from build123d import *

# Parameters (mm, degrees)
F0_R     = 3.175
F0_W     = 1.2134287943
F0_H     = 4.4488144882
F1_DEPTH = 3.048


with BuildPart() as f1:
    # F0 (on Front) → F1 (new body)
    with BuildSketch(Plane.XZ):
        with BuildLine():
            ThreePointArc((44.7334821429, -7.9324362036), (50.1620069047, -5.5115227815), (52.3875, 0))
            ThreePointArc((52.3875, 0), (50.1620069047, 5.5115227815), (44.7334821429, 7.9324362036))
            ThreePointArc((44.7334821429, 7.9324362036), (36.5125, 0), (44.7334821429, -7.9324362036))
        make_face()
        with Locations((44.45, 0)):
            Circle(F0_R, mode=Mode.SUBTRACT)
        with BuildLine():
            ThreePointArc((44.7334821429, -7.9324362036), (36.5125, 0), (44.7334821429, 7.9324362036))
            Line((44.7334821429, 7.9324362036), (18.9676000005, 8.8532337108))
            ThreePointArc((18.9676000005, 8.8532337108), (13.2611998974, 11.5713591498), (11.3411865923, 17.5933818124))
            Line((11.3411865923, 17.5933818124), (15.7954255641, 61.9125))
            ThreePointArc((15.7954255641, 61.9125), (0, 47.625), (-15.7954255641, 61.9125))
            Line((-15.7954255641, 61.9125), (-9.4772553384, -0.9525))
            ThreePointArc((-9.4772553384, -0.9525), (-0.4768479324, 9.5130563464), (9.525, 0))
            ThreePointArc((9.525, 0), (6.8544082857, -6.6138273378), (0.3401785714, -9.5189234444))
            Line((0.3401785714, -9.5189234444), (44.7334821429, -7.9324362036))
        make_face()
        with BuildLine():
            add(Edge.make_bspline(
                [(-4.1992530573, 32.2494809549), (-4.5608624776, 32.1718113259), (-5.0829042464, 32.1718113259)],
                knots=[0, 0, 0, 1, 1, 1], degree=2))
            add(Edge.make_bspline(
                [(-5.0829042464, 32.1718113259), (-6.156273054, 32.1718113259), (-6.7610775422, 32.7651563606)],
                knots=[0, 0, 0, 1, 1, 1], degree=2))
            add(Edge.make_bspline(
                [(-6.7610775422, 32.7651563606), (-7.3658820304, 33.3585013954), (-7.3658820304, 34.444602929)],
                knots=[0, 0, 0, 1, 1, 1], degree=2))
            add(Edge.make_bspline(
                [(-7.3658820304, 34.444602929), (-7.3658820304, 35.5625362778), (-6.806915356, 36.1730704928)],
                knots=[0, 0, 0, 1, 1, 1], degree=2))
            add(Edge.make_bspline(
                [(-6.806915356, 36.1730704928), (-6.2479486816, 36.7836047077), (-5.2611624114, 36.7836047077)],
                knots=[0, 0, 0, 1, 1, 1], degree=2))
            add(Edge.make_bspline(
                [(-5.2611624114, 36.7836047077), (-4.3189406823, 36.7836047077), (-3.793715732, 36.246920304)],
                knots=[0, 0, 0, 1, 1, 1], degree=2))
            add(Edge.make_bspline(
                [(-3.793715732, 36.246920304), (-3.2684907817, 35.7102359002), (-3.2684907817, 34.7629210807)],
                knots=[0, 0, 0, 1, 1, 1], degree=2))
            Line((-3.2684907817, 34.7629210807), (-3.2684907817, 34.1733958638))
            Line((-3.2684907817, 34.1733958638), (-6.1371739649, 34.1733958638))
            add(Edge.make_bspline(
                [(-6.1371739649, 34.1733958638), (-6.1168016031, 33.6564471854), (-5.8303152666, 33.3661410311)],
                knots=[0, 0, 0, 1, 1, 1], degree=2))
            add(Edge.make_bspline(
                [(-5.8303152666, 33.3661410311), (-5.5438289301, 33.0758348767), (-5.0268802517, 33.0758348767)],
                knots=[0, 0, 0, 1, 1, 1], degree=2))
            add(Edge.make_bspline(
                [(-5.0268802517, 33.0758348767), (-4.624526108, 33.0758348767), (-4.2667365054, 33.1592342324)],
                knots=[0, 0, 0, 1, 1, 1], degree=2))
            add(Edge.make_bspline(
                [(-4.2667365054, 33.1592342324), (-3.9089469029, 33.2426335882), (-3.5193254852, 33.4259848436)],
                knots=[0, 0, 0, 1, 1, 1], degree=2))
            Line((-3.5193254852, 33.4259848436), (-3.5193254852, 32.4863096597))
            add(Edge.make_bspline(
                [(-3.5193254852, 32.4863096597), (-3.8376436369, 32.3271505839), (-4.1992530573, 32.2494809549)],
                knots=[0, 0, 0, 1, 1, 1], degree=2))
        make_face(mode=Mode.SUBTRACT)
        with BuildLine():
            add(Edge.make_bspline(
                [(-0.5646964011, 36.5550522748), (-0.2126365253, 36.7836047077), (0.2011770719, 36.7836047077)],
                knots=[0, 0, 0, 1, 1, 1], degree=2))
            add(Edge.make_bspline(
                [(0.2011770719, 36.7836047077), (0.4481919576, 36.7836047077), (0.6111708513, 36.7479530748)],
                knots=[0, 0, 0, 1, 1, 1], degree=2))
            Line((0.6111708513, 36.7479530748), (0.5194952236, 35.6109206369))
            add(Edge.make_bspline(
                [(0.5194952236, 35.6109206369), (0.3717956012, 35.6503920877), (0.1617056211, 35.6503920877)],
                knots=[0, 0, 0, 1, 1, 1], degree=2))
            add(Edge.make_bspline(
                [(0.1617056211, 35.6503920877), (-0.4189066876, 35.6503920877), (-0.7435912024, 35.3518096614)],
                knots=[0, 0, 0, 1, 1, 1], degree=2))
            add(Edge.make_bspline(
                [(-0.7435912024, 35.3518096614), (-1.0682757171, 35.0532272351), (-1.0682757171, 34.515906195)],
                knots=[0, 0, 0, 1, 1, 1], degree=2))
            Line((-1.0682757171, 34.515906195), (-1.0682757171, 32.2520275001))
            Line((-1.0682757171, 32.2520275001), (-2.2817045114, 32.2520275001))
            Line((-2.2817045114, 32.2520275001), (-2.2817045114, 36.7008419883))
            Line((-2.2817045114, 36.7008419883), (-1.3624016893, 36.7008419883))
            Line((-1.3624016893, 36.7008419883), (-1.1828702517, 35.9521576955))
            Line((-1.1828702517, 35.9521576955), (-1.1242997118, 35.9521576955))
            add(Edge.make_bspline(
                [(-1.1242997118, 35.9521576955), (-0.9167562769, 36.3264998419), (-0.5646964011, 36.5550522748)],
                knots=[0, 0, 0, 1, 1, 1], degree=2))
        make_face(mode=Mode.SUBTRACT)
        with Locations((2.0251400811, 34.4764347442)):
            Rectangle(F0_W, F0_H, mode=Mode.SUBTRACT)
        with BuildLine():
            add(Edge.make_bspline(
                [(6.4694981152, 32.2437512281), (6.16900578, 32.1718113259), (5.7119009142, 32.1718113259)],
                knots=[0, 0, 0, 1, 1, 1], degree=2))
            add(Edge.make_bspline(
                [(5.7119009142, 32.1718113259), (3.6351932925, 32.1718113259), (3.6351932925, 34.4522425647)],
                knots=[0, 0, 0, 1, 1, 1], degree=2))
            add(Edge.make_bspline(
                [(3.6351932925, 34.4522425647), (3.6351932925, 35.5867284573), (4.1998896936, 36.1851665825)],
                knots=[0, 0, 0, 1, 1, 1], degree=2))
            add(Edge.make_bspline(
                [(4.1998896936, 36.1851665825), (4.7645860947, 36.7836047077), (5.8188558132, 36.7836047077)],
                knots=[0, 0, 0, 1, 1, 1], degree=2))
            add(Edge.make_bspline(
                [(5.8188558132, 36.7836047077), (6.5904590129, 36.7836047077), (7.2041764094, 36.4818390999)],
                knots=[0, 0, 0, 1, 1, 1], degree=2))
            Line((7.2041764094, 36.4818390999), (6.8451135342, 35.5421639161))
            add(Edge.make_bspline(
                [(6.8451135342, 35.5421639161), (6.5586271977, 35.6580317233), (6.3122489483, 35.7318815345)],
                knots=[0, 0, 0, 1, 1, 1], degree=2))
            add(Edge.make_bspline(
                [(6.3122489483, 35.7318815345), (6.0658706989, 35.8057313457), (5.8188558132, 35.8057313457)],
                knots=[0, 0, 0, 1, 1, 1], degree=2))
            add(Edge.make_bspline(
                [(5.8188558132, 35.8057313457), (4.8715409937, 35.8057313457), (4.8715409937, 34.4598822003)],
                knots=[0, 0, 0, 1, 1, 1], degree=2))
            add(Edge.make_bspline(
                [(4.8715409937, 34.4598822003), (4.8715409937, 33.1547777783), (5.8188558132, 33.1547777783)],
                knots=[0, 0, 0, 1, 1, 1], degree=2))
            add(Edge.make_bspline(
                [(5.8188558132, 33.1547777783), (6.16900578, 33.1547777783), (6.4675882063, 33.2483633149)],
                knots=[0, 0, 0, 1, 1, 1], degree=2))
            add(Edge.make_bspline(
                [(6.4675882063, 33.2483633149), (6.7661706326, 33.3419488515), (7.0641164226, 33.5418526508)],
                knots=[0, 0, 0, 1, 1, 1], degree=2))
            Line((7.0641164226, 33.5418526508), (7.0641164226, 32.5028622036))
            add(Edge.make_bspline(
                [(7.0641164226, 32.5028622036), (6.7699904504, 32.3156911304), (6.4694981152, 32.2437512281)],
                knots=[0, 0, 0, 1, 1, 1], degree=2))
        make_face(mode=Mode.SUBTRACT)
        with BuildLine():
            add(Edge.make_bspline(
                [(2.0270499901, 37.2534422997), (1.3662215071, 37.2534422997), (1.3662215071, 37.8506071523)],
                knots=[0, 0, 0, 1, 1, 1], degree=2))
            add(Edge.make_bspline(
                [(1.3662215071, 37.8506071523), (1.3662215071, 38.443952187), (2.0270499901, 38.443952187)],
                knots=[0, 0, 0, 1, 1, 1], degree=2))
            add(Edge.make_bspline(
                [(2.0270499901, 38.443952187), (2.687878473, 38.443952187), (2.687878473, 37.8506071523)],
                knots=[0, 0, 0, 1, 1, 1], degree=2))
            add(Edge.make_bspline(
                [(2.687878473, 37.8506071523), (2.687878473, 37.5679406335), (2.5229896704, 37.4106914666)],
                knots=[0, 0, 0, 1, 1, 1], degree=2))
            add(Edge.make_bspline(
                [(2.5229896704, 37.4106914666), (2.3581008678, 37.2534422997), (2.0270499901, 37.2534422997)],
                knots=[0, 0, 0, 1, 1, 1], degree=2))
        make_face(mode=Mode.SUBTRACT)
        with BuildLine():
            ThreePointArc((-9.4772553384, -0.9525), (-6.2623833816, -7.1769199091), (0.3401785714, -9.5189234444))
            ThreePointArc((0.3401785714, -9.5189234444), (6.8544082857, -6.6138273378), (9.525, 0))
            ThreePointArc((9.525, 0), (-0.4768479324, 9.5130563464), (-9.4772553384, -0.9525))
        make_face()
        Circle(F0_R, mode=Mode.SUBTRACT)
        with BuildLine():
            ThreePointArc((-15.7954255641, 61.9125), (0, 47.625), (15.7954255641, 61.9125))
            ThreePointArc((15.7954255641, 61.9125), (15.8550939106, 62.7052534459), (15.875, 63.5))
            ThreePointArc((15.875, 63.5), (15.8438414904, 64.4941387366), (15.7504882737, 65.484375))
            ThreePointArc((15.7504882737, 65.484375), (0, 79.375), (-15.7504882737, 65.484375))
            ThreePointArc((-15.7504882737, 65.484375), (-15.8737438155, 63.6997054867), (-15.7954255641, 61.9125))
        make_face()
        with Locations((0, 63.5)):
            Circle(F0_R, mode=Mode.SUBTRACT)
        with BuildLine():
            Line((-9.4502929642, 115.490625), (-15.7504882737, 65.484375))
            ThreePointArc((-15.7504882737, 65.484375), (0, 79.375), (15.7504882737, 65.484375))
            Line((15.7504882737, 65.484375), (9.4502929642, 115.490625))
            ThreePointArc((9.4502929642, 115.490625), (9.5063048942, 114.896483242), (9.525, 114.3))
            ThreePointArc((9.525, 114.3), (-0.596483242, 104.7936951058), (-9.4502929642, 115.490625))
        make_face()
        with Locations((-3.175, 100.0252)):
            Circle(F0_R, mode=Mode.SUBTRACT)
        with BuildLine():
            ThreePointArc((9.4502929642, 115.490625), (0, 123.825), (-9.4502929642, 115.490625))
            ThreePointArc((-9.4502929642, 115.490625), (-0.596483242, 104.7936951058), (9.525, 114.3))
            ThreePointArc((9.525, 114.3), (9.5063048942, 114.896483242), (9.4502929642, 115.490625))
        make_face()
        with Locations((0, 114.3)):
            Circle(F0_R, mode=Mode.SUBTRACT)
    extrude(amount=F1_DEPTH)


solid = f1.part
Could you check a few things on this model? Use its own coordinates, in mm. A direction names the side the tool comes from. Round coordinates to 2 decimals unless told otherwise and drop trailing zeros. Order: outer loops, then holes, each group sorted by start corner. A loop starts at its lowest first (then second) coordinate and runs counter-clockwise, first axis right, second up. Notation, with made-up numbers: M 81,-8 L 120,-8 A27 cw 120,29 Z; hole C 16.5,58.5 d7. An arc over 180 degrees is marked long. One line per item, written item: value.
(1) If we mould it in two halves opening along X, with no side actions, what happens to faces 1 (the flat face through (-12.68, -1.5, 30.92)), 2 (the flat face through (3, 0, 43)), 3 (the flat face through (-1.068, -2, 33))? For each: released by +X, released by -X, zero draft, split by the parting line, or undercut.
Ans:
face 1: released by -X
face 2: zero draft
face 3: undercut
(2) Imagine slicing it at C-C (x = 27). Write out the boundary of the cut face in (y, z), and give its area (3 significant figures).
Ans:
outline: M -3.05,-8.57 L 0,-8.57 L 0,8.57 L -3.05,8.57 Z
area: 52.2 mm^2
(3) I'm going to push flat-ended pins straight in: P1, Ø7.5, axis at x = 44.45, z = 0, coming from the +Y side; P2, Ø0.5, axis at x = -2, y = -2, coming from the -Z side; P3, Ø0.6, axis at x = 1.5, y = -1.5, coming from the +Z side; P4, Ø1.1, axis at y = -1, z = 33, coming from the -X side. Where does each tip first touch, or does it pass through?
Ans:
P1: stops at y = 0
P2: stops at z = -9.36
P3: stops at z = 123.75
P4: stops at x = -12.94
(4) Imagine slicing it at B-B (z = 25). Write out the boundary of the cut face in (x, y), and give its area (3 significant figures).
Ans:
outline: M -12.09,-3.05 L 12.09,-3.05 L 12.09,0 L -12.09,0 Z
area: 73.7 mm^2
(5) Which directions (+Z, -Z, +X, -X, +Y, -Y) give clear straight access to the entire face, cutting with the end or side of a thin tool? Please do faces 4 (the cylindrical face through (-15.873, -1.503, 63.725)), 5 (the flat face through (13.537, -1.503, 39.443)), 6 (the flat face through (2.632, -2, 34)).
Ans:
face 4: -X, +Y, -Y
face 5: +X, +Y, -Y
face 6: +Y, -Y
(6) Imagine slicing it at A-A (x = 42.5). Write out the boundary of the cut face in (y, z).
Ans:
outline: M -3.05,-8.01 L 0,-8.01 L 0,-2.51 L -3.05,-2.51 Z; M -3.05,2.51 L 0,2.51 L 0,8.01 L -3.05,8.01 Z
(7) I need wall thicknesses on line 1 along Z through (x, y) = (1, -0.3); line 2 along X through (y, z) = (-1.45, 52); line 3 along X through (y, z) = (-2.4, 43.5). Which ranges of each line are inside material? Lowest first, please. Write a range as from..to.
Ans:
line 1: z = -9.5..-3.01, 3.01..60.49, 66.51..111.29, 117.31..123.77
line 2: x = -14.8..14.8
line 3: x = -13.94..13.94
(8) Imagine slicing it at D-D (y = -2.15). Count the separate pieces of the cut face and the enclosed holes in it, and give its area (3 significant figures).
Ans:
separate pieces: 1
enclosed holes: 10
area: 3,740 mm^2
